For this review, take the finished solid that the model builds, in its own axes (mm). A direction names the side the tool comes from. Give positions to 0.01 mm unless a question says otherwise; leave off trailing zeros. Write each loop counter-clockwise with the first axis right and the second up, starting at its lowest first coordinate (ties: lowest second). Pieces come first, ordered by that corner, then holes.
1) Draft analysis for pull direction Y (two halves, no side actions). For faces 1 (the face through (-27, 18, 40)), 2 (the face through (-18.34, 5.93, 27.96)), 3 (the face through (-56, 16.99, 20)), state which applies: pulls with the +Y half, pulls with the -Y half, needs draft (parallel to the pull), parting line crosses it, or undercut.
2) Wall thickness on line 1 along X through (y, z) = (12.5, 30); line 2 along X through (y, z) = (10, 12.5); line 3 along Y through (x, z) = (-43, 33): over which ranges is each line inside the solid? List them lowest first.
3) For P1, Ø4.5, axis at x = -50, z = 24.5, coming from the -Y side; P2, Ø3.5, axis at x = -56.5, z = 25.5, coming from the -Y side; P3, Ø1.8, axis at x = -14, z = 19, coming from the -Y side, all flat-tipped, find the tip position at first contact; note any pin that passes through.
4) We need section A-A on x = -12. Give the boundary of the cut face in (y, z), and give its area (3 significant figures).
5) We need section C-C on z = 21. Give the boundary of the cut face in (x, y), and give its area (4 significant figures).
6) We need section D-D on y = 5.5. Give the boundary of the cut face in (x, z).
7) We need section B-B on z = 30. Give the number of separate pieces and of enclosed holes in the cut face, and give its area (3 significant figures).
8) Machinability: for faces 4 (the face through (-16.315, 7, 20)), 5 (the face through (-53.815, 14, 20)), 6 (the face through (-10.787, 5.074, 31.757)), which of the approach directions +Z, -Z, +X, -X, +Y, -Y give a long, thin tool a straight path to every point of the face, cutting with its end or side? Answer none if there is none.
from build123d import *

# Parameters (mm, degrees)
F0_W           = 4
F0_H           = 20
F0_W_2         = 6
F0_H_2         = 5.5
F1_DEPTH       = 40
F2_SIZE        = 1
F4_D           = 4.6
F4_DEPTH       = 12
F4_CBORE_D     = 5.2
F4_CBORE_DEPTH = 6


with BuildPart() as f1:
    # F0 (on Top) → F1 (new body)
    with BuildSketch(Plane.XY):
        Polygon((-8.815112, 20.990383), (-58.815112, 20.990383), (-58.815112, 16.990383), (-53.815112, 16.990383), (-47.815112, 16.990383), (-20.315112, 16.990383), (-16.315112, 16.990383), (-12.815112, 16.990383), (-8.815112, 16.990383), align=None)
        with Locations((-10.815112, 6.990383)):
            Rectangle(F0_W, F0_H)
        with Locations((-50.815112, 14.240383)):
            Rectangle(F0_W_2, F0_H_2)
        with Locations((-18.315112, 6.990383)):
            Rectangle(F0_W, F0_H)
    extrude(amount=F1_DEPTH)

    # F2
    f2_edges = [f1.edges().sort_by_distance(p)[0] for p in [
        (-47.815112, 16.990383, 20),
        (-53.815112, 16.990383, 20),
        (-53.815112, 11.490383, 20),
        (-58.815112, 16.990383, 20),
        (-58.815112, 20.990383, 20),
        (-8.815112, 20.990383, 20),
        (-8.815112, -3.009617, 20),
        (-33.815112, 20.990383, 40),
        (-33.815112, 20.990383, 0),
        (-20.315112, 16.990383, 20),
        (-8.815112, 8.990383, 40),
        (-8.815112, 8.990383, 0),
        (-58.815112, 18.990383, 40),
        (-58.815112, 18.990383, 0),
        (-47.815112, 11.490383, 20),
        (-10.815112, -3.009617, 0),
        (-10.815112, -3.009617, 40),
    ]]
    chamfer(f2_edges, length=F2_SIZE)

    # F4
    with Locations(Plane.YZ.offset(-8.815112)):
        with Locations((6.990383, 10), (6.990383, 30)):
            CounterBoreHole(F4_D / 2, F4_CBORE_D / 2, F4_CBORE_DEPTH, depth=F4_DEPTH)


solid = f1.part
Results list:
1. face 1: needs draft
1. face 2: undercut
1. face 3: pulls with the -Y half
2. line 1: x = -53.82 to -47.82, -20.32 to -16.32, -12.82 to -8.82
2. line 2: x = -20.32 to -16.32, -12.82 to -8.82
2. line 3: y = 16.99 to 20.99
3. P1: stops at y = 11.49
3. P2: stops at y = 16.93
3. P3: stops at y = 16.99
4. outline: (-3.01, 1) - (-2.01, 0) - (19.99, 0) - (20.99, 1) - (20.99, 39) - (19.99, 40) - (-2.01, 40) - (-3.01, 39) - close; hole circle Ø5.2 at (6.99, 10); hole circle Ø5.2 at (6.99, 30)
4. area: 916 mm2
5. outline: (-58.82, 17.99) - (-57.82, 16.99) - (-54.82, 16.99) - (-53.82, 15.99) - (-53.82, 12.49) - (-52.82, 11.49) - (-48.82, 11.49) - (-47.82, 12.49) - (-47.82, 15.99) - (-46.82, 16.99) - (-21.32, 16.99) - (-20.32, 15.99) - (-20.32, -3.01) - (-16.32, -3.01) - (-16.32, 16.99) - (-12.82, 16.99) - (-12.82, -3.01) - (-9.82, -3.01) - (-8.82, -2.01) - (-8.82, 19.99) - (-9.82, 20.99) - (-57.82, 20.99) - (-58.82, 19.99) - close
5. area: 391.5 mm2
6. outline: (-20.32, 0) - (-16.32, 0) - (-16.32, 8.25) - (-20.32, 8.25) - close; (-20.32, 11.75) - (-16.32, 11.75) - (-16.32, 28.25) - (-20.32, 28.25) - close; (-20.32, 31.75) - (-16.32, 31.75) - (-16.32, 40) - (-20.32, 40) - close; (-12.82, 0) - (-9.82, 0) - (-8.82, 1) - (-8.82, 7.87) - (-12.82, 7.87) - close; (-12.82, 12.13) - (-8.82, 12.13) - (-8.82, 27.87) - (-12.82, 27.87) - close; (-12.82, 32.13) - (-8.82, 32.13) - (-8.82, 39) - (-9.82, 40) - (-12.82, 40) - close
7. separate pieces: 3
7. enclosed holes: 0
7. area: 352 mm2
8. face 4: +Z, -Z, -Y
8. face 5: +Z, -Z, -X, -Y
8. face 6: +X
